Geometry check sheet. Reference: the model listing, model coordinates, mm. Face numbers are marked on the shaded views. A direction names the side the tool comes from. Give positions to 0.01 mm unless a question says otherwise; leave off trailing zeros. Write each loop counter-clockwise with the first axis right and the second up, starting at its lowest first coordinate (ties: lowest second). Pieces come first, ordered by that corner, then holes. Notation, with made-up numbers: (88.25, 71) - (129.25, 71) arc R32 cw to (129.25, 98) - close; hole circle Ø4 at (-25.5, 13.5). An arc over 180 degrees is marked (long way). One line per question, with ' | ' between items. Start each with the question number.
Q1. Section check B-B on y = -17. Record the boundary of the cut face in (x, z).
Q2. Thickness scan on L1, parallel to Y at x = 0.75, z = -21.25; L2, parallel to Z at x = 1, y = -23; L3, parallel to Y at x = -10, z = -6. Record the ranges inside material, lowest first. Write a range as [from, to].
Q3. Set-up check for the marked faces 1 and 2: record each of +Z, -Z, +X, -X, +Y, -Y from which the full face is reachable in a straight line by a thin tool's end or side.
Q4. Release check for a two-part mould opening along Z. For the marked faces 3, 4 and 5 record: +Z half, -Z half, draft (parallel to the pull), parting line (faces both ways), or undercut.
Q5. Section check A-A on y = -9.25. Record the boundary of the cut face in (x, z), and give its area (3 significant figures).
Q6. Section check C-C on x = -4. Record the boundary of the cut face in (y, z).
Q7. Section check D-D on z = -5.25. Count the separate pieces of the cut face and the enclosed holes in it, and give its area (3 significant figures).
Q8. Gauge pin test, flat ends, axial feed: P1, Ø13, axis at x = -16.5, z = -17.5, coming from the +Y side; P2, Ø5, axis at y = -31, z = -21.5, coming from the -X side; P3, Ø6, axis at y = -10, z = -18, coming from the -X side. Record the tip position at first contact, or that the pin passes through.
```python
from build123d import *

# Parameters (mm, degrees)
SKETCH_1_W      = 26.5
SKETCH_1_H      = 32.5
SKETCH_1_R      = 5
SKETCH_1_R_2    = 1.65
EXTRUDE_1_DEPTH = 2.8
SKETCH_3_R      = 3.9
SKETCH_3_R_2    = 1.65
EXTRUDE_2_DEPTH = 2.8
FILLET_2_R      = 3
FILLET_3_R      = 3
FILLET_4_R      = 2
FILLET_5_R      = 2


with BuildPart() as part:
    # 草图1 → 凸台-拉伸1 (new body)
    with BuildSketch(Plane(origin=(0, 0, 0), x_dir=(0, 0, -1), z_dir=(1, 0, 0))):
        with Locations((13.25, -16.25)):
            Rectangle(SKETCH_1_W, SKETCH_1_H)
        with Locations((13.25, -16.25)):
            Circle(SKETCH_1_R, mode=Mode.SUBTRACT)
        with Locations((5.25, -9.25)):
            Circle(SKETCH_1_R_2, mode=Mode.SUBTRACT)
        with Locations((21.25, -9.25)):
            Circle(SKETCH_1_R_2, mode=Mode.SUBTRACT)
        with Locations((5.25, -23.25)):
            Circle(SKETCH_1_R_2, mode=Mode.SUBTRACT)
        with Locations((21.25, -23.25)):
            Circle(SKETCH_1_R_2, mode=Mode.SUBTRACT)
    extrude(amount=EXTRUDE_1_DEPTH)

    # 草图3 → 凸台-拉伸2 (add)
    with BuildSketch(Plane.XZ.offset(32.5)):
        with BuildLine():
            Line((2.8, 0), (-17.2, 0))
            ThreePointArc((-17.2, 0), (-30.45, -13.25), (-17.2, -26.5))
            Line((-17.2, -26.5), (2.8, -26.5))
            Line((2.8, -26.5), (2.8, 0))
        make_face()
        with Locations(Location((-17.2, -13.25, 0), (0, 0, 270))):
            Circle(SKETCH_3_R, mode=Mode.SUBTRACT)
        with Locations(Location((-17.2, -4.75, 0), (0, 0, 270))):
            Circle(SKETCH_3_R_2, mode=Mode.SUBTRACT)
        with Locations(Location((-17.2, -21.75, 0), (0, 0, 90))):
            Circle(SKETCH_3_R_2, mode=Mode.SUBTRACT)
    extrude(amount=EXTRUDE_2_DEPTH)

    # 圆角2
    fillet_2_edges = [part.edges().sort_by_distance(p)[0] for p in [
        (1.4, 0, -26.5),
    ]]
    fillet(fillet_2_edges, radius=FILLET_2_R)

    # 圆角3
    fillet_3_edges = [part.edges().sort_by_distance(p)[0] for p in [
        (1.4, 0, 0),
    ]]
    fillet(fillet_3_edges, radius=FILLET_3_R)

    # 圆角4
    fillet_4_edges = [part.edges().sort_by_distance(p)[0] for p in [
        (2.8, -35.3, -13.25),
    ]]
    fillet(fillet_4_edges, radius=FILLET_4_R)

    # 圆角5
    fillet_5_edges = [part.edges().sort_by_distance(p)[0] for p in [
        (-30.45, -35.3, -13.25),
        (-8.2, -35.3, -26.5),
        (2.8, 0, -13.25),
        (2.8, -0.878679656, -25.621320344),
        (2.8, -18.15, 0),
        (2.8, -0.878679656, -0.878679656),
        (-8.2, -35.3, 0),
        (2.214213562, -34.714213562, 0),
        (2.8, -18.15, -26.5),
        (2.214213562, -34.714213562, -26.5),
    ]]
    fillet(fillet_5_edges, radius=FILLET_5_R)


solid = part.part
```
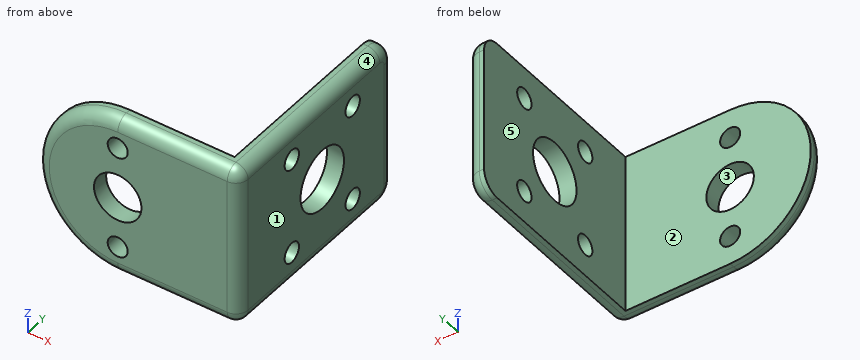
Working result:
1) outline: (0, -26.5) - (0.8, -26.5) arc R2 ccw to (2.8, -24.5) - (2.8, -18.19) - (0, -18.19) - close; (0, -8.31) - (2.8, -8.31) - (2.8, -2) arc R2 ccw to (0.8, 0) - (0, 0) - close
2) L1: y = [-35.3, -24.9], [-21.6, -10.9], [-7.6, 0] | L2: z = [-26.49, -22.88], [-19.62, -6.88], [-3.62, -0.01] | L3: y = [-35.3, -32.5]
3) face 1: +Z, -Z, +X, +Y, -Y | face 2: +Z, -Z, -X, +Y
4) face 3: undercut | face 4: +Z half | face 5: draft
5) outline: (0, -26.5) - (0.8, -26.5) arc R2 ccw to (2.8, -24.5) - (2.8, -22.9) - (0, -22.9) - close; (0, -19.6) - (2.8, -19.6) - (2.8, -6.9) - (0, -6.9) - close; (0, -3.6) - (2.8, -3.6) - (2.8, -2) arc R2 ccw to (0.8, 0) - (0, 0) - close | area: 54.0 mm2
6) outline: (-35.3, -24.5) arc R2 ccw to (-33.3, -26.5) - (-32.5, -26.5) - (-32.5, 0) - (-33.3, 0) arc R2 ccw to (-35.3, -2) - close
7) separate pieces: 4 | enclosed holes: 0 | area: 146 mm2
8) P1: stops at y = -32.5 | P2: stops at x = -28.88 | P3: stops at x = 0
